```python
from build123d import *

# Parameters (mm, degrees)
SKETCH_1_R               = 7.5
SKETCH_1_R_2             = 1.5
SKETCH_1_R_3             = 2
EXTRUDE_1_DEPTH          = 5
EXTRUDE_2_DEPTH          = 5
CUT_EXTRUDE_1_DEPTH      = 55.790510127
CUT_EXTRUDE_1_DEPTH_BACK = 55.790510127
SKETCH_4_W               = 18.755882419
SKETCH_4_H               = 70
CUT_EXTRUDE_2_DEPTH      = 55.790510127
CUT_EXTRUDE_2_DEPTH_BACK = 55.790510127
SKETCH_5_R               = 1.5
CUT_EXTRUDE_3_DEPTH      = 55.790510127
CUT_EXTRUDE_3_DEPTH_BACK = 55.790510127
SKETCH_7_R               = 1.5
SKETCH_8_R               = 3
CUT_EXTRUDE_4_DEPTH      = 1.7


with BuildPart() as part:
    # 草图1 → 凸台-拉伸1 (new body)
    with BuildSketch(Plane(origin=(0, 0, 0), x_dir=(1, 0, 0), z_dir=(0, 1, 0))):
        with BuildLine():
            Line((0, 36), (38, 36))
            ThreePointArc((38, 36), (40.121320344, 35.121320344), (41, 33))
            Line((41, 33), (41, -33))
            ThreePointArc((41, -33), (40.121320344, -35.121320344), (38, -36))
            Line((38, -36), (0, -36))
            ThreePointArc((0, -36), (-36, 0), (0, 36))
        make_face()
        with Locations(Location((0, 0, 0), (0, 0, 270))):
            Circle(SKETCH_1_R, mode=Mode.SUBTRACT)
        with Locations(Location((-6.783865663, 11.75, 0), (0, 0, 270))):
            Circle(SKETCH_1_R_2, mode=Mode.SUBTRACT)
        with Locations(Location((6.783865663, 11.75, 0), (0, 0, 270))):
            Circle(SKETCH_1_R_2, mode=Mode.SUBTRACT)
        with Locations(Location((13.567731326, 0, 0), (0, 0, 270))):
            Circle(SKETCH_1_R_2, mode=Mode.SUBTRACT)
        with Locations(Location((6.783865663, -11.75, 0), (0, 0, 270))):
            Circle(SKETCH_1_R_2, mode=Mode.SUBTRACT)
        with Locations(Location((-6.783865663, -11.75, 0), (0, 0, 270))):
            Circle(SKETCH_1_R_2, mode=Mode.SUBTRACT)
        with Locations(Location((-13.567731326, 0, 0), (0, 0, 270))):
            Circle(SKETCH_1_R_2, mode=Mode.SUBTRACT)
        with Locations(Location((-12, -6.92820323, 0), (0, 0, 270))):
            Circle(SKETCH_1_R_3, mode=Mode.SUBTRACT)
        with Locations(Location((0, 13.856406461, 0), (0, 0, 270))):
            Circle(SKETCH_1_R_3, mode=Mode.SUBTRACT)
        with Locations(Location((12, -6.92820323, 0), (0, 0, 270))):
            Circle(SKETCH_1_R_3, mode=Mode.SUBTRACT)
    extrude(amount=EXTRUDE_1_DEPTH)

    # 草图3 → 凸台-拉伸2 (add)
    with BuildSketch(Plane(origin=(0, 5, 0), x_dir=(1, 0, 0), z_dir=(0, 1, 0))):
        with BuildLine():
            Line((0, 36), (-34.75, 36))
            Line((-34.75, 36), (-35.75, 35))
            Line((-35.75, 35), (-35.75, -35))
            Line((-35.75, -35), (-34.75, -36))
            Line((-34.75, -36), (0, -36))
            ThreePointArc((0, -36), (-34.929573093, 0), (0, 36))
        make_face()
    extrude(amount=-EXTRUDE_2_DEPTH)

    # 草图4 → 切除-拉伸1 (cut, two sides: drawn at the far end of the back side and taken through both)
    with BuildSketch(Plane.XZ.offset(-CUT_EXTRUDE_1_DEPTH_BACK)):
        with Locations((-45.12794121, 0)):
            Rectangle(SKETCH_4_W, SKETCH_4_H)
    extrude(amount=CUT_EXTRUDE_1_DEPTH + CUT_EXTRUDE_1_DEPTH_BACK, mode=Mode.SUBTRACT)

    # 草图5 → 切除-拉伸2 (cut, two sides: drawn at the far end of the back side and taken through both)
    with BuildSketch(Plane(origin=(0, 5, 0), x_dir=(1, 0, 0), z_dir=(0, 1, 0)).offset(-CUT_EXTRUDE_2_DEPTH_BACK)):
        with Locations(Location((-7.125, -31, 0), (0, 0, 270))):
            Circle(SKETCH_5_R)
        with Locations(Location((-32.875, -31, 0), (0, 0, 270))):
            Circle(SKETCH_5_R)
        with Locations(Location((-7.125, 31, 0), (0, 0, 270))):
            Circle(SKETCH_5_R)
        with Locations(Location((-32.875, 31, 0), (0, 0, 270))):
            Circle(SKETCH_5_R)
    extrude(amount=CUT_EXTRUDE_2_DEPTH + CUT_EXTRUDE_2_DEPTH_BACK, mode=Mode.SUBTRACT)

    # 草图7 → 切除-拉伸3 (cut, two sides: drawn at the far end of the back side and taken through both)
    with BuildSketch(Plane.XZ.offset(-CUT_EXTRUDE_3_DEPTH_BACK)):
        with Locations(Location((37.8, -32.8, 0), (0, 0, 270))):
            Circle(SKETCH_7_R)
        with Locations(Location((19.2, -31.3, 0), (0, 0, 270))):
            Circle(SKETCH_7_R)
        with Locations(Location((33.412894333, 5.952122667, 0), (0, 0, 270))):
            Circle(SKETCH_7_R)
        with Locations(Location((37.8, 32.8, 0), (0, 0, 270))):
            Circle(SKETCH_7_R)
        with Locations(Location((19.2, 31.3, 0), (0, 0, 270))):
            Circle(SKETCH_7_R)
    extrude(amount=CUT_EXTRUDE_3_DEPTH + CUT_EXTRUDE_3_DEPTH_BACK, mode=Mode.SUBTRACT)

    # 草图8 → 切除-拉伸4 (cut)
    with BuildSketch(Plane.XZ):
        with Locations(Location((-7.125, 31, 0), (0, 0, 270))):
            Circle(SKETCH_8_R)
        with Locations(Location((-7.125, -31, 0), (0, 0, 270))):
            Circle(SKETCH_8_R)
    extrude(amount=-CUT_EXTRUDE_4_DEPTH, mode=Mode.SUBTRACT)


solid = part.part
```
Model file for the job. Use its own axes, mm. A direction names the side the tool comes from. Round coordinates to 2 decimals unless told otherwise and drop trailing zeros. Order: outer loops, then holes, each group sorted by start corner. A loop starts at its lowest first (then second) coordinate and runs counter-clockwise, first axis right, second up. Notation, with made-up numbers: M 33.5,-34 L 76.5,-34 A35 cw 76.5,4 Z; hole C 41,-25.75 d4. An arc over 180 degrees is marked long. Use CSV: the item, a comma, the result in double quotes.
Item 1: Saw through at B-B (x = 19.2). List the corners of the cut face in (y, z), plus the area to 3 significant figures.
Worked answers:
outline,"M 0,-36 L 5,-36 L 5,-32.8 L 0,-32.8 Z; M 0,-29.8 L 5,-29.8 L 5,29.8 L 0,29.8 Z; M 0,32.8 L 5,32.8 L 5,36 L 0,36 Z"
area,"330 mm²"
Item 2: Probe probe 1 along Z at (x, y) = (19.2, 2.1); probe 2 along Z at (x, y) = (37.8, 3.05); probe 3 along X at (y, z) = (1.7, 0). List the from-to ranges inside material, lowest first.
Worked answers:
probe 1,"-36 to -32.8, -29.8 to 29.8, 32.8 to 36"
probe 2,"-36 to -34.3, -31.3 to 31.3, 34.3 to 36"
probe 3,"-35.75 to -15.07, -12.07 to -7.5, 7.5 to 12.07, 15.07 to 41"
Item 3: Pull direction X, two halves, no side cores. Call faces 3 (the face through (-35.75, 3, 0)), 4 (the face through (40.14, 2.46, 35.1)), 5 (the face through (-15.03, 2.46, -0.33)): released by +X, released by -X, zero draft, split by the parting line, or undercut.
Worked answers:
face 3,"released by -X"
face 4,"released by +X"
face 5,"undercut"
Item 4: Saw through at C-C (y = 3.6). State how many separate pieces and enclosed holes the cut face has, plus the area to 3 significant figures.
Worked answers:
separate pieces,"1"
enclosed holes,"19"
area,"5,200 mm²"
Item 5: Saw through at A-A (z = 0). List the corners of the cut face in (x, y), plus the area to 3 significant figures.
Worked answers:
outline,"M -35.75,0 L -15.07,0 L -15.07,5 L -35.75,5 Z; M -12.07,0 L -7.5,0 L -7.5,5 L -12.07,5 Z; M 7.5,0 L 12.07,0 L 12.07,5 L 7.5,5 Z; M 15.07,0 L 41,0 L 41,5 L 15.07,5 Z"
area,"279 mm²"
Item 6: Pin check, flat tip, straight feed: pin 1 (2.5 mm diameter, centred on x = -6.78, z = 11.75, fed in from -Y). Stop position of the tip, or through.
Worked answers:
pin 1,"through"
Item 7: Which spindle directions (+Z, -Z, +X, -X, +Y, -Y) get a long thin tool onto all of the face, cutting with end or side? Do faces 1 (the face through (2, 0, -9)), 2 (the face through (-6.993, 0.838, -28.003)). Say none if no direction does.
Worked answers:
face 1,"+Z, -Z, +X, -X, -Y"
face 2,"-Y"
